from build123d import *

# Parameters (mm, degrees)
F0_W      = 14.25
F0_H      = 37.5
F0_R      = 1.625
F0_R_2    = 1.5
F1_DEPTH  = 6.5
F2_R      = 1.175
F3_DEPTH  = 5.5
F4_R      = 0.635
F5_W      = 3
F5_H      = 6.75
F6_DEPTH  = 14
F7_W      = 24.5
F7_H      = 4.325
F8_DEPTH  = 4
F9_W      = 13.4
F9_H      = 1.5
F10_DEPTH = 2
F10_TAPER = 15
F12_DEPTH = 4
F13_R     = 1.27


with BuildPart() as f1:
    # F0 (on Front) → F1 (new body)
    with BuildSketch(Plane.XZ):
        with Locations((-7.125, 18.75)):
            Rectangle(F0_W, F0_H)
        with Locations((-7.125, 15.35)):
            Circle(F0_R, mode=Mode.SUBTRACT)
        with Locations((-7.125, 23.425)):
            Circle(F0_R_2, mode=Mode.SUBTRACT)
        with Locations((-7.125, 31.5)):
            Circle(F0_R, mode=Mode.SUBTRACT)
        with Locations((-7.125, 23.425)):
            Circle(F0_R_2)
    extrude(amount=F1_DEPTH)

    # F2 (on face) → F3 (join)
    with BuildSketch(Plane(origin=(0, 0, 0), x_dir=(-1, 0, 0), z_dir=(0, 1, 0))):
        with Locations((7.125, 23.425)):
            Circle(F2_R)
    extrude(amount=F3_DEPTH)

    # F4
    f4_edges = [f1.edges().sort_by_distance(p)[0] for p in [
        (-5.95, 5.5, 23.425),
    ]]
    fillet(f4_edges, radius=F4_R)

    # F5 (on face) → F6 (cut)
    with BuildSketch(Plane(origin=(-14.25, 0, 0), x_dir=(0, -1, 0), z_dir=(-1, 0, 0))):
        with Locations((3.25, 31.5)):
            Rectangle(F5_W, F5_H)
        with Locations((3.25, 15.35)):
            Rectangle(F5_W, F5_H)
    extrude(amount=-F6_DEPTH, mode=Mode.SUBTRACT)

    # F7 (on face) → F8 (cut)
    with BuildSketch(Plane.XZ.offset(6.5)):
        with Locations((-7.125, 2.1625)):
            Rectangle(F7_W, F7_H)
    extrude(amount=-F8_DEPTH, mode=Mode.SUBTRACT)

    # F9 (on face) → F10 (join)
    with BuildSketch(Plane.XZ.offset(2.5)):
        with Locations((-7.125, 0.75)):
            Rectangle(F9_W, F9_H)
        with Locations((-7.125, 3.25)):
            Rectangle(F9_W, F9_H)
    extrude(amount=F10_DEPTH, taper=F10_TAPER)

    # F11 (on face) → F12 (cut)
    with BuildSketch(Plane(origin=(0, 0, 0), x_dir=(1, 0, 0), z_dir=(0, 0, -1))):
        Polygon((-14.25, 4.8693548888), (-14.25, 2.5), (-13.825, 2.5), (-12.125, 4.5109390723), (-2.125, 4.5109390723), (-0.425, 2.5), (0, 2.5), (0, 4.8693548888), align=None)
    extrude(amount=-F12_DEPTH, mode=Mode.SUBTRACT)

    # F13
    f13_edges = [f1.edges().sort_by_distance(p)[0] for p in [
        (-7.125, -6.5, 4.325),
        (-14.25, -6.5, 20.9125),
        (0, -6.5, 20.9125),
    ]]
    fillet(f13_edges, radius=F13_R)


solid = f1.part
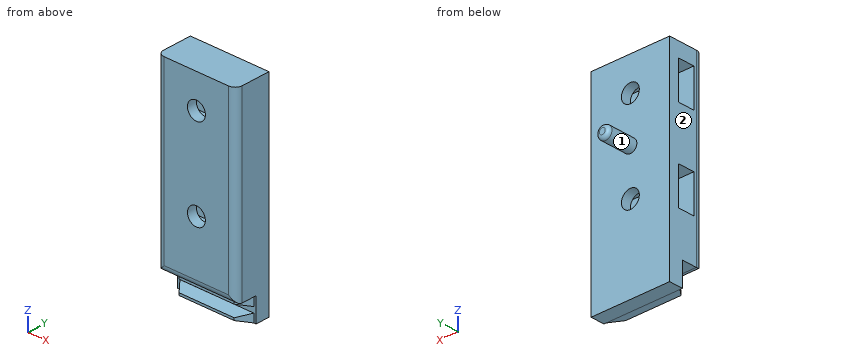
Input: part model. Units: mm. Frame: model coordinates. Face numbers are marked on the shaded views. A direction names the side the tool comes from. Round coordinates to 2 decimals unless told otherwise and drop trailing zeros. Order: outer loops, then holes, each group sorted by start corner. A loop starts at its lowest first (then second) coordinate and runs counter-clockwise, first axis right, second up. Notation, with made-up numbers: (83, 2) - (113, 2) arc R28 ccw to (113, 30) - close; hole circle Ø3 at (-8.75, 50.5). An arc over 180 degrees is marked (long way). Answer as a JSON object with one key per item and string values. Group by question number.
(1) Reachability of the marked faces 1 and 2 from +Z, -Z, +X, -X, +Y, -Y: full face, straight path, thin tool, end or side. Return the list, or none.
(2) Cut plane B-B (x = -10.5). Count the separate pieces of the cut face and the enclosed holes in it, then the cut area to 3 significant figures.
(3) Material intervals for probe 1 along Y at (x, z) = (-11.5, 33.5); probe 2 along Z at (x, y) = (-7.5, -5.5); probe 3 along X at (y, z) = (-5.3, 31.5), sorted ascending. Write a range as from..to.
(4) Cut plane C-C (z = 14.5). Return loops of the section in (x, y).
(5) Cut plane D-D (z = 10). Return loops of the section in (x, y), then the cut area to 3 significant figures.
(6) Cut plane A-A (z = 31.5). Return loops of the section in (x, y).
(7) Pin query (flat end, axial travel): P1, Ø7.5, axis at x = -6.5, z = 16.5, coming from the +Y side; P2, Ø1.5, axis at y = -3, z = 32.5, coming from the -X side. Return the tip coordinate at first contact, or that it passes through.
Here are the results:
{
 "1": {"face 1": "+Y", "face 2": "+Z, -Z, -X, +Y, -Y"},
 "2": {"separate pieces": "1", "enclosed holes": "2", "area": "189 mm^2"},
 "3": {"probe 1": "y = -6.5..-4.75, -1.75..0", "probe 2": "z = 4.35..13.77, 16.93..29.92, 33.08..37.5", "probe 3": "x = -14.25..-8.75, -5.5..0"},
 "4": {"outline": "(-14.25, -5.23) arc R1.27 ccw to (-12.98, -6.5) - (-8.51, -6.5) - (-8.51, -4.75) - (-14.25, -4.75) - close; (-14.25, -1.75) - (-8.51, -1.75) - (-8.51, 0) - (-14.25, 0) - close; (-5.74, -6.5) - (-1.27, -6.5) arc R1.27 ccw to (0, -5.23) - (0, 0) - (-5.74, 0) - (-5.74, -1.75) - (-0.25, -1.75) - (-0.25, -4.75) - (-5.74, -4.75) - close"},
 "5": {"outline": "(-14.25, -5.23) arc R1.27 ccw to (-12.98, -6.5) - (-1.27, -6.5) arc R1.27 ccw to (0, -5.23) - (0, 0) - (-14.25, 0) - close", "area": "91.9 mm^2"},
 "6": {"outline": "(-14.25, -5.23) arc R1.27 ccw to (-12.98, -6.5) - (-8.75, -6.5) - (-8.75, -4.75) - (-14.25, -4.75) - close; (-14.25, -1.75) - (-8.75, -1.75) - (-8.75, 0) - (-14.25, 0) - close; (-5.5, -6.5) - (-1.27, -6.5) arc R1.27 ccw to (0, -5.23) - (0, 0) - (-5.5, 0) - (-5.5, -1.75) - (-0.25, -1.75) - (-0.25, -4.75) - (-5.5, -4.75) - close"},
 "7": {"P1": "stops at y = 0", "P2": "stops at x = -0.25"}
}
